from build123d import *

# Parameters (mm, degrees)
SKETCH021_W     = 2
SKETCH021_H     = 54
PAD012_DEPTH    = 20
POCKET007_DEPTH = 2
SKETCH023_R     = 2
POCKET008_DEPTH = 2
SKETCH024_W     = 29
SKETCH024_H     = 8.5
POCKET009_DEPTH = 2


with BuildPart() as part:
    # Sketch021 → Pad012 (new body)
    with BuildSketch(Plane.XY.offset(20)):
        with Locations((52, 0)):
            Rectangle(SKETCH021_W, SKETCH021_H)
    extrude(amount=-PAD012_DEPTH)

    # Sketch022 (on Face4 of Pad012) → Pocket007 (cut)
    with BuildSketch(Plane.YZ.offset(53)):
        with BuildLine():
            Line((-19, 3.999999), (-19, 8))
            ThreePointArc((-19, 8), (-21, 10), (-23, 7.999999))
            Line((-23, 3.999999), (-23, 7.999999))
            ThreePointArc((-23, 3.999999), (-21, 2), (-19, 3.999999))
        make_face()
    extrude(amount=-POCKET007_DEPTH, mode=Mode.SUBTRACT)

    # Sketch023 (on Face2 of Pocket007) → Pocket008 (cut)
    with BuildSketch(Plane.YZ.offset(53)):
        with Locations((21, 8)):
            Circle(SKETCH023_R)
    extrude(amount=-POCKET008_DEPTH, mode=Mode.SUBTRACT)

    # Sketch024 (on Face2 of Pocket008) → Pocket009 (cut)
    with BuildSketch(Plane.YZ.offset(53)):
        with Locations((0, 5.75)):
            Rectangle(SKETCH024_W, SKETCH024_H)
    extrude(amount=-POCKET009_DEPTH, mode=Mode.SUBTRACT)


solid = part.part
For this review, take the finished solid that the model builds, in its own axes (mm). A direction names the side the tool comes from. Give positions to 0.01 mm unless a question says otherwise; leave off trailing zeros. Loops run counter-clockwise (first coordinate to the right, second up) from the corner with the lowest first, then second, coordinate; pieces in that order, holes last. Notation, with made-up numbers: M -4,85.25 L 39,85.25 A16 cw 39,105.25 Z; hole C 74.25,12.5 d9. An arc over 180 degrees is marked long. Answer as a JSON object with one key per item and string values. Group by question number.
Q1. Mouldability with a two-part tool opening along Z and no side actions: class faces 3 (the cylindrical face through (52.014, 19.526, 9.352)), 4 (the flat face through (52, 0, 0)), 5 (the flat face through (52, 0, 1.5)), 6 (the flat face through (51, 0, 12)) as +Z half, -Z half, draft (parallel to the pull), parting line (faces both ways), or undercut.
Q2. Add section B-B on x = 52.4. Give the boundary of the cut face in (y, z), and give its area (3 significant figures).
Q3. For probe 1 along Z at (x, y) = (52.55, 21); probe 2 along Y at (x, z) = (51.4, 2.5); probe 3 along Y at (x, z) = (51.2, 6.25), list the stretches that pass through material, from the lowest coordinate up. Write a range as [from, to].
Q4. Add section D-D on y = -14. Give the boundary of the cut face in (x, z), and give its area (3 significant figures).
Q5. Add section C-C on z = 5. Give the boundary of the cut face in (x, y), and give its area (3 significant figures).
Q6. Tool access review of faces 1 (the flat face through (52, -23, 6)), 2 (the flat face through (52, -27, 10)): name each direction out of +Z, -Z, +X, -X, +Y, -Y from which nothing blocks a thin tool from reaching the whole face with its end or side.
Q7. Add section A-A on y = -21. Give the boundary of the cut face in (x, z).
Checked values:
{
 "1": {"face 3": "undercut", "face 4": "-Z half", "face 5": "undercut", "face 6": "draft"},
 "2": {"outline": "M -27,0 L 27,0 L 27,20 L -27,20 Z; hole M -23,4 A2 ccw -19,4 L -19,8 A2 ccw -23,8 Z; hole M -14.5,1.5 L 14.5,1.5 L 14.5,10 L -14.5,10 Z; hole C 21,8 d4", "area": "792 mm²"},
 "3": {"probe 1": "[0, 6], [10, 20]", "probe 2": "[-27, -22.32], [-19.68, -14.5], [14.5, 27]", "probe 3": "[-27, -23], [-19, -14.5], [14.5, 20.03], [21.97, 27]"},
 "4": {"outline": "M 51,0 L 53,0 L 53,1.5 L 51,1.5 Z; M 51,10 L 53,10 L 53,20 L 51,20 Z", "area": "23.0 mm²"},
 "5": {"outline": "M 51,-27 L 53,-27 L 53,-23 L 51,-23 Z; M 51,-19 L 53,-19 L 53,-14.5 L 51,-14.5 Z; M 51,14.5 L 53,14.5 L 53,27 L 51,27 Z", "area": "42.0 mm²"},
 "6": {"face 1": "+X, -X", "face 2": "+Z, -Z, +X, -X, -Y"},
 "7": {"outline": "M 51,0 L 53,0 L 53,2 L 51,2 Z; M 51,10 L 53,10 L 53,20 L 51,20 Z"}
}
